from build123d import *

# Parameters (mm, degrees)
SKETCH1_W               = 15
SKETCH1_H               = 25.4
BOSS_EXTRUDE1_DEPTH     = 3.175
CUT_EXTRUDE1_DEPTH      = 22.305369042
CUT_EXTRUDE1_DEPTH_BACK = 22.305369042
SKETCH2_W               = 3
SKETCH2_H               = 12.5
FILLET1_R               = 1.5


with BuildPart() as part:
    # Sketch1 → Boss-Extrude1 (new body)
    with BuildSketch(Plane(origin=(0, 0, 0), x_dir=(1, 0, 0), z_dir=(0, 1, 0))):
        Polygon((-7.5, -12.7), (-7.5, 12.7), (-7.5, 15.875), (-13.85, 15.875), (-13.85, -15.875), (-7.5, -15.875), align=None)
        Rectangle(SKETCH1_W, SKETCH1_H)
    extrude(amount=BOSS_EXTRUDE1_DEPTH)

    # Sketch2 → Cut-Extrude1 (cut, two sides: drawn at the far end of the back side and taken through both)
    with BuildSketch(Plane(origin=(0, 3.175, 0), x_dir=(1, 0, 0), z_dir=(0, 1, 0)).offset(-CUT_EXTRUDE1_DEPTH_BACK)):
        with Locations((1.5875, 0)):
            Rectangle(SKETCH2_W, SKETCH2_H)
    extrude(amount=CUT_EXTRUDE1_DEPTH + CUT_EXTRUDE1_DEPTH_BACK, mode=Mode.SUBTRACT)

    # Fillet1
    fillet1_edges = [part.edges().sort_by_distance(p)[0] for p in [
        (3.0875, 1.5875, -6.25),
        (3.0875, 1.5875, 6.25),
        (0.0875, 1.5875, 6.25),
        (0.0875, 1.5875, -6.25),
    ]]
    fillet(fillet1_edges, radius=FILLET1_R - 0.0001)  # a hair under: the kernel refuses the full size


solid = part.part
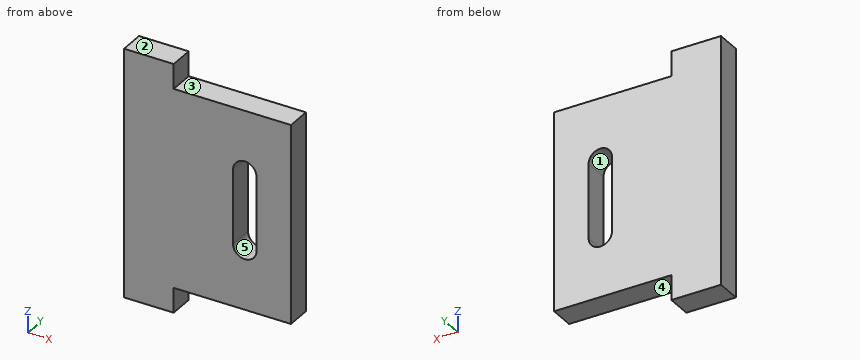
Check sheet for the modelled part. Datum: model origin and axes. Units: mm. Face numbers are marked on the shaded views. A direction names the side the tool comes from. Coordinates: 2 decimals unless noted, no trailing zeros. Loops run counter-clockwise (first coordinate to the right, second up) from the corner with the lowest first, then second, coordinate; pieces in that order, holes last. Notation, with made-up numbers: (-32, 34.25) -> (0, 34.25) arc R19 cw to (0, 53.25) -> close; hole circle Ø1 at (30.25, -24). An arc over 180 degrees is marked (long way). Write item = value, one per line. Start each with the question number.
1. Section check D-D on x = -6. Record the cut outline in (y, z) (3 decimals), then the cut area to 3 significant figures.
2. Material ranges on line 1 (X direction, y = 0.7, z = 3.5); line 2 (Z direction, x = -0.5, y = 2.4); line 3 (X direction, y = 0.8, z = -13.5), recorded low to high.
3. Depth check by flat-ended pin: P1, Ø1.6, axis at y = 2, z = 14, coming from the +X side; P2, Ø1, axis at x = 2.5, y = 0.5, coming from the -Z side. Enter the tip coordinate at first touch or a pass-through.
4. Tool access check on the marked faces 1, 2 and 3. Record the directions out of +Z, -Z, +X, -X, +Y, -Y that give a thin tool (end or side, any length) a straight path to the whole face; none if there is none.
5. Draft check along X on the marked faces 4 and 5. Enter one of: released by +X, released by -X, zero draft, split by the parting line, or undercut.
6. Section check C-C on x = 2. Record the cut outline in (y, z) (3 decimals), then the cut area to 3 significant figures.
Responses:
q1.outline = (0, -12.7) -> (3.175, -12.7) -> (3.175, 12.7) -> (0, 12.7) -> close
q1.area = 80.6 mm2
q2.line_1 = -13.85 to 0.09, 3.09 to 7.5
q2.line_2 = -12.7 to 12.7
q2.line_3 = -13.85 to -7.5
q3.P1 = -7.5
q3.P2 = -12.7
q4.face_1 = +Y, -Y
q4.face_2 = +Z, +X, -X, +Y, -Y
q4.face_3 = +Z, +X, +Y, -Y
q5.face_4 = zero draft
q5.face_5 = undercut
q6.outline = (0, -12.7) -> (3.175, -12.7) -> (3.175, -6.192) -> (0, -6.192) -> close; (0, 6.192) -> (3.175, 6.192) -> (3.175, 12.7) -> (0, 12.7) -> close
q6.area = 41.3 mm2
